Geometry check sheet. Reference: the model listing, model coordinates, mm. Round coordinates to 2 decimals unless told otherwise and drop trailing zeros. Loops run counter-clockwise (first coordinate to the right, second up) from the corner with the lowest first, then second, coordinate; pieces in that order, holes last. Notation, with made-up numbers: M 82.25,59 L 135.25,59 A12 ccw 135.25,66 Z; hole C -30,57 d1. An arc over 180 degrees is marked long. Write item = value, one per line.
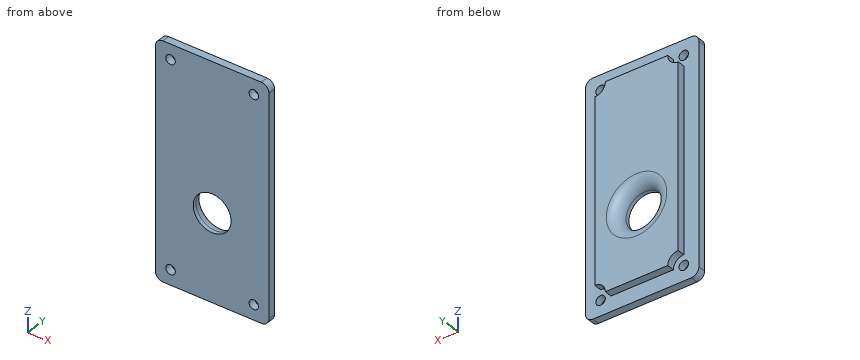
Autodesk Inventor part; units mm, degrees
ref_plane "YZ Plane" through (0, 0, 0) normal (1, 0, 0) x (0, 1, 0)
ref_plane "XZ Plane" through (0, 0, 0) normal (0, 1, 0) x (-1, 0, 0)
ref_plane "XY Plane" through (0, 0, 0) normal (0, 0, 1) x (1, 0, 0)
sketch "스케치1" plane through (0, 0, 0) normal (0, 1, 0) x (-1, 0, 0)
  line L0 (11, 27) -> (-11, 27)
  line L1 (-11, 27) -> (-11, -27)
  line L2 (-11, -27) -> (11, -27)
  line L3 (11, -27) -> (11, 27)
  line L4 (11, 27) -> (-11, -27) construction
  line L5 (-11, 27) -> (11, -27) construction
  line L6 (15, 31) -> (-15, 31)
  line L7 (-15, 31) -> (-15, -31)
  line L8 (-15, -31) -> (15, -31)
  line L9 (15, -31) -> (15, 31)
  circle A0 centre (11, 27) radius 1.25
  line L10 (0, 0) -> (0, -5.338)
  line L11 (0, 0) -> (0.8274, 0)
  line L12 (0, 0) -> (4.4604, 0)
  circle A1 centre (11, 27) radius 2.75
  circle A2 centre (11, -27) radius 1.25
  circle A3 centre (11, -27) radius 2.75
  circle A4 centre (-11, 27) radius 1.25
  circle A5 centre (-11, 27) radius 2.75
  circle A6 centre (-11, -27) radius 1.25
  circle A7 centre (-11, -27) radius 2.75
  point P0 (-11, -24.25)
  point P1 (-8.25, -27)
  point P2 (8.25, -27)
  point P3 (11, -24.25)
  point P4 (11, 24.25)
  point P5 (8.25, 27)
  point P6 (-8.25, 27)
  point P7 (-11, 24.25)
  dimension "d0" = 22
  dimension "d1" = 54
  dimension "d2" = 4
  dimension "d3" = 2.5
  dimension "d4" = 5.5
extrude "돌출1" add sketch "스케치1" against normal blind 2 contours A5 L1 A4 L0 | L0 A4 L1 A5 | L0 A1 L3 A3 L2 A7 L1 A5 | A1 L3 A0 L0 | L0 A0 L3 A1 | A7 L2 A6 L1 | L1 A6 L2 A7 | A3 L2 A2 L3 | L3 A2 L2 A3 | L9 L8 L7 L6
extrude "돌출2" add sketch "스케치1" along normal blind 2 contours L0 A1 L3 A3 L2 A7 L1 A5
fillet "모깎기1" radius 2 4 edges at (15, -1, -31) (-15, -1, -31) (15, -1, 31) (-15, -1, 31)
sketch "스케치2" plane through (0, 2, 0) normal (0, 1, 0) x (1, 0, 0)
  circle A0 centre (0, 8) radius 5
  line L0 (13, 31) -> (-13, 31)
  point P0 (0, 0)
  dimension "d10" = 23
  dimension "d11" = 10
extrude "돌출3" cut sketch "스케치2" against normal blind 4
fillet "모깎기2" radius 3 1 edges at (-5, 2, -8)
properties part number "커튼 서보 커버"
(1) Sectioned sample at B-B on x = 0. Record the cut outline in (y, z).
Result set:
outline = M -2,-31 L 0,-31 L 0,-27 L 2,-27 L 2,-16 A3 ccw -1,-13 L -2,-13 Z; M -2,-3 L -1,-3 A3 ccw 2,0 L 2,27 L 0,27 L 0,31 L -2,31 Z
(2) Material ranges on line 1 along X through (y, z) = (-0.9, 27); line 2 along Z through (x, y) = (11, -1.4); line 3 along X through (y, z) = (-1.3, -8), recorded low to high. Write a range as from..to.
Result set:
line_1 = -15..-12.25, -9.75..9.75, 12.25..15
line_2 = -31..-28.25, -25.75..25.75, 28.25..31
line_3 = -15..-5, 5..15
(3) Sectioned sample at A-A on z = -8. Record the cut outline in (x, y), then the cut area to 3 significant figures.
Result set:
outline = M -15,-2 L -5,-2 L -5,-1 A3 ccw -8,2 L -11,2 L -11,0 L -15,0 Z; M 5,-2 L 15,-2 L 15,0 L 11,0 L 11,2 L 8,2 A3 ccw 5,-1 Z
area = 60.1 mm2
(4) Sectioned sample at D-D on z = 9. Record the cut outline in (x, y).
Result set:
outline = M -15,-2 L 15,-2 L 15,0 L 11,0 L 11,2 L -11,2 L -11,0 L -15,0 Z
(5) Depth check by flat-ended pin: pin 1 Ø15 at (x, z) = (0, -5) entering from +Y; pin 2 Ø1.5 at (x, z) = (-11, -27) entering from -Y; pin 3 Ø1 at (x, y) = (2.5, 1.5) entering from -Z; pin 4 Ø0.6 at (x, y) = (-0.5, 1) entering from +Z. Enter the tip coordinate at first touch or a pass-through.
Result set:
pin_1 = 2
pin_2 = through
pin_3 = -27
pin_4 = 27
(6) Sectioned sample at C-C on y = 1.4. Record the cut outline in (x, z).
Result set:
outline = M -11,-24.25 A2.75 cw -8.25,-27 L 8.25,-27 A2.75 cw 11,-24.25 L 11,24.25 A2.75 cw 8.25,27 L -8.25,27 A2.75 cw -11,24.25 Z; hole C 0,-8 d12.4
